```python
from build123d import *

# Parameters (mm, degrees)
SKETCH_W   = 90
SKETCH_H   = 160
SKETCH_R   = 1.5
SKETCH_W_2 = 7
SKETCH_H_2 = 32
PAD_DEPTH  = 3


with BuildPart() as part:
    # Sketch → Pad (new body)
    with BuildSketch(Plane.XY):
        with Locations((45, 80)):
            Rectangle(SKETCH_W, SKETCH_H)
        with Locations((10, 155)):
            Circle(SKETCH_R, mode=Mode.SUBTRACT)
        with Locations((10, 105)):
            Circle(SKETCH_R, mode=Mode.SUBTRACT)
        with Locations((27.5, 139.05)):
            Circle(SKETCH_R, mode=Mode.SUBTRACT)
        with Locations((45.5, 139.05)):
            Circle(SKETCH_R, mode=Mode.SUBTRACT)
        with Locations((27.5, 120.95)):
            Circle(SKETCH_R, mode=Mode.SUBTRACT)
        with Locations((45.5, 120.95)):
            Circle(SKETCH_R, mode=Mode.SUBTRACT)
        with Locations((4, 156.75)):
            Circle(SKETCH_R, mode=Mode.SUBTRACT)
        with Locations((16, 156.75)):
            Circle(SKETCH_R, mode=Mode.SUBTRACT)
        with Locations((4, 103.25)):
            Circle(SKETCH_R, mode=Mode.SUBTRACT)
        with Locations((16, 103.25)):
            Circle(SKETCH_R, mode=Mode.SUBTRACT)
        with Locations((10, 130)):
            Rectangle(SKETCH_W_2, SKETCH_H_2, mode=Mode.SUBTRACT)
    pad = extrude(amount=PAD_DEPTH)

    # Mirrored: Pad across face of Pad
    add(pad.mirror(Plane(origin=(90, 80, 1.5), x_dir=(0, 1, 0), z_dir=(1, 0, 0))))


solid = part.part
```
Check sheet for the modelled part. Datum: model origin and axes. Units: mm. Coordinates: 2 decimals unless noted, no trailing zeros. One line per question, with ' | ' between items. Start each with the question number.
Item 1: Material ranges on line 1 (X direction, y = 156.75, z = 0.65); line 2 (X direction, y = 126, z = 2.1); line 3 (X direction, y = 155, z = 0.95), recorded low to high.
Item 2: Gauge pin test, flat end, axial feed: P1, Ø2.5, axis at x = 10, y = 105, coming from the -Z side. Record the tip position at first contact, or that the pin passes through.
Item 3: Sectioned sample at A-A on z = 2. Count the separate pieces of the cut face and the enclosed holes in it, and give its area (3 significant figures).
Answer below:
1) line 1: x = 0 to 2.5, 5.5 to 14.5, 17.5 to 162.5, 165.5 to 174.5, 177.5 to 180 | line 2: x = 0 to 6.5, 13.5 to 166.5, 173.5 to 180 | line 3: x = 0 to 8.5, 11.5 to 168.5, 171.5 to 180
2) P1: passes through
3) separate pieces: 1 | enclosed holes: 22 | area: 28,200 mm^2
